Part print with two shaded views. Sizes in mm from the minimum x, y, z corner. Coordinates: 2 decimals unless noted, no trailing zeros. Write each question's results on one line, items separated by ' | '. Start each with the question number.
Q1. Wall check: probe 1 along X at (y, z) = (9.5, 3.25) (1 decimal); probe 2 along X at (y, z) = (10.5, 6.75); probe 3 along Y at (x, z) = (24, 3.75) (1 decimal). Give the ranges that are in metal, low to high.
Q2. Pull direction Y, two halves, no side cores. Call the marked faces 1, 2 and 3: released by +Y, released by -Y, zero draft, split by the parting line, or undercut.
Q3. Pin check, flat tips, straight feed: P1, Ø5, axis at x = 16.5, y = 9, coming from the -Z side; P2, Ø1, axis at x = 27, z = 5.5, coming from the +Y side; P3, Ø1.5, axis at y = 25.5, z = 6.5, coming from the +X side. Stop position of each tip, or through.
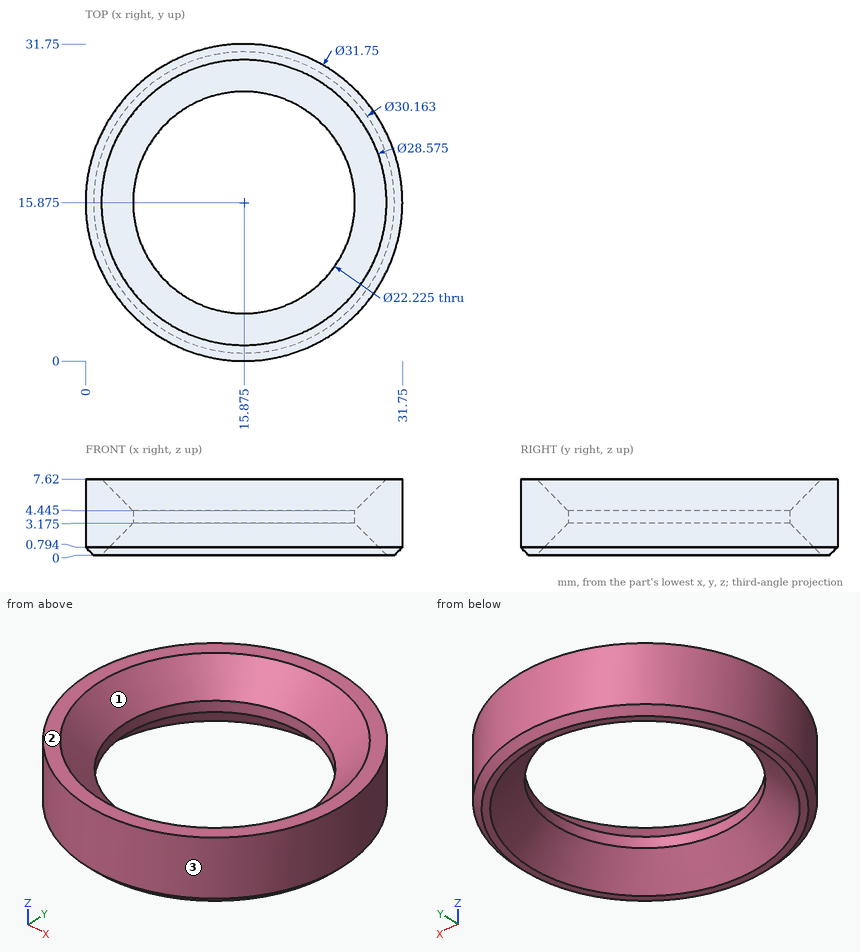
Results below:
1) probe 1: x = 1.3 to 6.8, 25 to 30.4 | probe 2: x = 0.94 to 3.58, 28.17 to 30.81 | probe 3: y = 2.2 to 8.3, 23.5 to 29.5
2) face 1: undercut | face 2: zero draft | face 3: split by the parting line
3) P1: passes through | P2: stops at y = 27.67 | P3: stops at x = 29.04
